The model under review builds one solid part; all positions refer to its coordinate system, in mm. A direction names the side the tool comes from. Coordinates: 2 decimals unless noted, no trailing zeros. Loops run counter-clockwise (first coordinate to the right, second up) from the corner with the lowest first, then second, coordinate; pieces in that order, holes last. Notation, with made-up numbers: M 68,52.5 L 115,52.5 A24 cw 115,91.5 Z; hole C 54,-35.5 d8. An arc over 180 degrees is marked long. Return JSON: item names as keys, results as strings.
```python
from build123d import *

# Parameters (mm, degrees)
ESQUISSE25_R = 1.9


with BuildPart() as part:
    # Balayage7: sweep along a path in Esquisse23
    with BuildLine(Plane.XY) as balayage7_path:
        Line((2, -5), (1, -5))
        ThreePointArc((1, -5), (0.292893219, -4.707106781), (0, -4))
        Line((0, -4), (0, -3))
        ThreePointArc((0, -3), (0.292893219, -2.292893219), (1, -2))
        Line((1, -2), (15, -2))
        ThreePointArc((15, -2), (15.707106781, -2.292893219), (16, -3))
        Line((16, -3), (16, -4))
        ThreePointArc((16, -4), (15.707106781, -4.707106781), (15, -5))
        Line((15, -5), (14, -5))
    # Esquisse25 → Balayage7 (sweep)
    with BuildSketch(Plane(origin=(2, 0, 0), x_dir=(0, 0, -1), z_dir=(1, 0, 0))):
        with Locations((0, -12.623519933)):
            Circle(ESQUISSE25_R)
    sweep(path=balayage7_path.line)


solid = part.part
```
1. The part is to be moulded in two halves that separate along X. For faces 3 (the face through (1.49, -13.91, 1.4)), 4 (the face through (14, -13, 0)), say which applies: released by +X, released by -X, zero draft, split by the parting line, or undercut.
Check values:
{"face 3": "undercut", "face 4": "undercut"}
2. Add section B-B on x = 2.5. Give the boundary of the cut face in (y, z), plus the area to 3 significant figures.
Check values:
{"outline": "C 5.62,0 d3.8", "area": "11.3 mm²"}
3. To check wall thickness, follow line 1 (Y direction, x = 0, z = -1.15); line 2 (X direction, y = -0.5, z = 1.65); line 3 (Y direction, x = -0.5, z = -0.1). State the ranges of each line that lie inside material, in increasing order.
Check values:
{"line 1": "-14.09 to -11.04, 4.04 to 7.09", "line 2": "-8.23 to -6.26, 22.26 to 24.23", "line 3": "-14.41 to -10.56, 3.56 to 7.41"}
4. Add section A-A on z = 0. Give the boundary of the cut face in (x, y).
Check values:
{"outline": "M -9.52,-4 A10.52 ccw 1,-14.52 L 2,-14.52 L 2,-10.72 L 1,-10.72 A6.72 cw -5.72,-4 L -5.72,-3 A6.72 cw 1,3.72 L 15,3.72 A6.72 cw 21.72,-3 L 21.72,-4 A6.72 cw 15,-10.72 L 14,-10.72 L 14,-14.52 L 15,-14.52 A10.52 ccw 25.52,-4 L 25.52,-3 A10.52 ccw 15,7.52 L 1,7.52 A10.52 ccw -9.52,-3 Z"}
5. Machinability: for faces 1 (the face through (21.77, -3.51, 0.41)), 2 (the face through (2, -13, 0)), which of the approach directions +Z, -Z, +X, -X, +Y, -Y give a long, thin tool a straight path to every point of the face, cutting with its end or side? Answer none if there is none.
Check values:
{"face 1": "none", "face 2": "+Z, -Z, -Y"}
6. Insertion check: pin 1 Ø4 at (x, y) = (19, -8.5) entering from +Z; pin 2 Ø1.9 at (y, z) = (-13.5, 0) entering from +X; pin 3 Ø2 at (y, z) = (5, 0) entering from +X. Each pin has a flat end and moves straight along its axis. Give the tip position at first contact, or say it passes through.
Check values:
{"pin 1": "z = 1.8", "pin 2": "x = 21.14", "pin 3": "x = 22.86"}
